Geometry: see drawing. Coordinates: mm, zero at the bounding-box minimum. A direction names the side the tool comes from. Round coordinates to 2 decimals unless told otherwise and drop trailing zeros. Loops run counter-clockwise (first coordinate to the right, second up) from the corner with the lowest first, then second, coordinate; pieces in that order, holes last. Notation, with made-up numbers: (-28, 22.5) - (18, 22.5) arc R29 ccw to (18, 47.5) - close; hole circle Ø1 at (-5.5, -4). An arc over 180 degrees is marked (long way). Write item = value, one per line. Start each with the question number.
Item 1: First-contact query: pin 1 (3 mm diameter, centred on x = 35, y = 50.5, fed in from -Z); pin 2 (4 mm diameter, centred on y = 77.5, z = 23.5, fed in from -X); pin 3 (2 mm diameter, centred on x = 13, y = 15.5, fed in from -Z); pin 4 (7.5 mm diameter, centred on y = 26, z = 9, fed in from -X). Flat tips, straight axial feed; report the tip coordinate or a pass-through.
Item 2: Draft query along X for the marked faces 1, 2 and 3. Return one class per face: pulls with the +X half, pulls with the -X half, needs draft (parallel to the pull), parting line crosses it, or undercut.
Item 3: Section B-B (x = 35). Return loops of the section in (y, z), plus the area to 3 significant figures.
Item 4: Line query: line 1 (Y direction, x = 35, z = 18.35); line 2 (Y direction, x = 8, z = 28.5); line 3 (X direction, y = 24, z = 17). Output: solid intervals per line, ascending. Write a range as from..to.
Item 5: Section A-A (y = 50.5). Return loops of the section in (x, z), plus the area to 3 significant figures.
Item 6: Access query for the marked faces 4, 5, 6 and 7. Directions: +Z, -Z, +X, -X, +Y, -Y. A direction counts if a zero-diameter tool reaches every point of the face in a straight line with its end or side. Return the directions, or none.
Item 7: Section D-D (z = 8). Return loops of the section in (x, y).
Item 8: Section C-C (z = 21.5). Return loops of the section in (x, y).
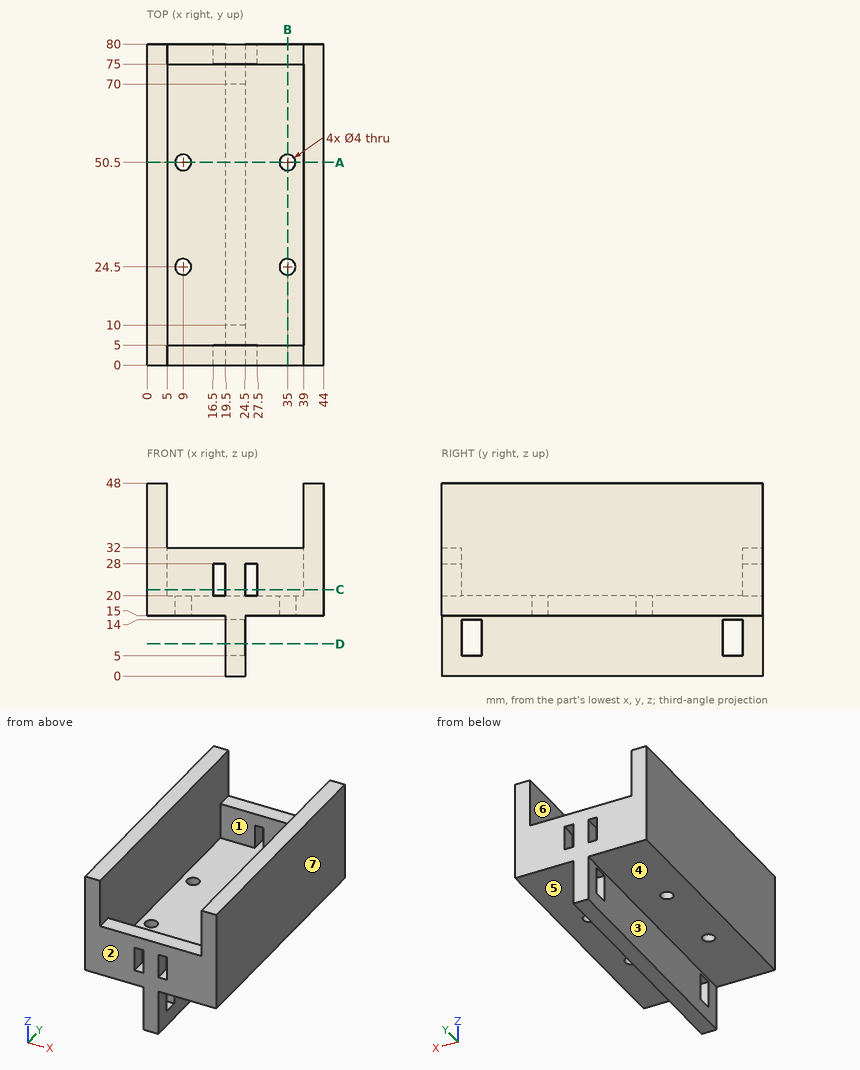
Taken from the geometry:
q1.pin_1 = through
q1.pin_2 = 0
q1.pin_3 = 15
q1.pin_4 = 19.5
q2.face_1 = undercut
q2.face_2 = needs draft
q2.face_3 = pulls with the -X half
q3.outline = (0, 15) - (22.5, 15) - (22.5, 20) - (5, 20) - (5, 32) - (0, 32) - close; (26.5, 15) - (48.5, 15) - (48.5, 20) - (26.5, 20) - close; (52.5, 15) - (80, 15) - (80, 32) - (75, 32) - (75, 20) - (52.5, 20) - close
q3.area = 480 mm^2
q4.line_1 = 0..22.5, 26.5..48.5, 52.5..80
q4.line_2 = 0..5, 75..80
q4.line_3 = 0..7.06, 10.94..33.06, 36.94..44
q5.outline = (0, 15) - (7, 15) - (7, 20) - (5, 20) - (5, 48) - (0, 48) - close; (11, 15) - (19.5, 15) - (19.5, 0) - (24.5, 0) - (24.5, 15) - (33, 15) - (33, 20) - (11, 20) - close; (37, 15) - (44, 15) - (44, 48) - (39, 48) - (39, 20) - (37, 20) - close
q5.area = 535 mm^2
q6.face_4 = -Z, -X, +Y, -Y
q6.face_5 = -Z, +X, +Y, -Y
q6.face_6 = +Z
q6.face_7 = +Z, -Z, +X, +Y, -Y
q7.outline = (19.5, 0) - (24.5, 0) - (24.5, 5) - (19.5, 5) - close; (19.5, 10) - (24.5, 10) - (24.5, 70) - (19.5, 70) - close; (19.5, 75) - (24.5, 75) - (24.5, 80) - (19.5, 80) - close
q8.outline = (0, 0) - (16.5, 0) - (16.5, 5) - (5, 5) - (5, 75) - (16.5, 75) - (16.5, 80) - (0, 80) - close; (19.5, 0) - (24.5, 0) - (24.5, 5) - (19.5, 5) - close; (19.5, 75) - (24.5, 75) - (24.5, 80) - (19.5, 80) - close; (27.5, 0) - (44, 0) - (44, 80) - (27.5, 80) - (27.5, 75) - (39, 75) - (39, 5) - (27.5, 5) - close
